```python
from build123d import *

# Parameters (mm, degrees)
SKETCH_W     = 33
SKETCH_H     = 50
SKETCH_R     = 3.25
PAD_DEPTH    = 3
FILLET_R     = 2
FILLET001_R  = 10
PAD001_DEPTH = 4.8
SKETCH002_R  = 1.25
POCKET_DEPTH = 8.001
CHAMFER_SIZE = 0.5


with BuildPart() as part:
    # Sketch → Pad (new body)
    with BuildSketch(Plane.XY):
        with Locations((16.5, 25)):
            Rectangle(SKETCH_W, SKETCH_H)
        with Locations((24, 41)):
            Circle(SKETCH_R, mode=Mode.SUBTRACT)
    extrude(amount=PAD_DEPTH)

    # Fillet
    fillet_edges = [part.edges().sort_by_distance(p)[0] for p in [
        (0, 0, 1.5),
    ]]
    fillet(fillet_edges, radius=FILLET_R)

    # Fillet001
    fillet001_edges = [part.edges().sort_by_distance(p)[0] for p in [
        (33, 0, 1.5),
        (0, 50, 1.5),
        (33, 50, 1.5),
    ]]
    fillet(fillet001_edges, radius=FILLET001_R)

    # Sketch001 → Pad001 (join)
    with BuildSketch(Plane.XY.offset(3)):
        Polygon((20, 22), (20, 27.5), (1, 27.5), (1, 22), (17, 22), (17, 21), (20, 21), align=None)
        Polygon((1, 0.5), (1, 6), (17, 6), (17, 7), (20, 7), (20, 6), (20, 0.5), align=None)
    extrude(amount=PAD001_DEPTH)

    # Sketch002 → Pocket (cut, through all)
    with BuildSketch(Plane.XY.offset(8)):
        with Locations((16, 24)):
            Circle(SKETCH002_R)
        with Locations((16, 4)):
            Circle(SKETCH002_R)
    extrude(amount=-POCKET_DEPTH, mode=Mode.SUBTRACT)

    # Chamfer
    chamfer_edges = [part.edges().sort_by_distance(p)[0] for p in [
        (9, 22, 7.8),
        (9, 6, 7.8),
        (17, 21.5, 7.8),
        (17, 6.5, 7.8),
        (18.5, 7, 7.8),
        (18.5, 21, 7.8),
    ]]
    chamfer(chamfer_edges, length=CHAMFER_SIZE)


solid = part.part
```
Can you work these out from the model? Positions are in its coordinate system, mm. A direction names the side the tool comes from. Coordinates: 2 decimals unless noted, no trailing zeros. Write each loop counter-clockwise with the first axis right and the second up, starting at its lowest first coordinate (ties: lowest second). Pieces come first, ordered by that corner, then holes. Notation, with made-up numbers: M -3.75,60 L 3.25,60 A22 ccw 3.25,97 Z; hole C 16,36 d11. An arc over 180 degrees is marked long. Answer as CSV lines item,"result".
Item 1: We'd pull the mould along X, two halves only. Please class faces 1 (the cylindrical face through (15.73, 2.78, 3.95)), 2 (the flat face through (0, 21, 1)), 3 (the cylindrical face through (29.99, 47.15, 1.52)): +X half, -X half, draft (parallel to the pull), parting line (faces both ways), or undercut.
Geometry results:
face 1,"undercut"
face 2,"-X half"
face 3,"+X half"
Item 2: Imagine slicing it at A-A on z = 5.25. List the corners of the cut face in (x, y) for me, plus the area to 3 significant figures.
Geometry results:
outline,"M 1,0.5 L 20,0.5 L 20,7 L 17,7 L 17,6 L 1,6 Z; M 1,22 L 17,22 L 17,21 L 20,21 L 20,27.5 L 1,27.5 Z; hole C 16,4 d2.5; hole C 16,24 d2.5"
area,"205 mm2"
Item 3: I'm going to push flat-ended pins straight in: P1, Ø2.5, axis at x = 18, z = 4.5, coming from the +Y side; P2, Ø0.5, axis at y = 6.5, z = 6, coming from the -X side; P3, Ø2.5, axis at y = 25.5, z = 4.5, coming from the +X side; P4, Ø4, axis at x = 24, y = 41, coming from the +Z side. Where does each tip first touch, or does it pass through?
Geometry results:
P1,"stops at y = 27.5"
P2,"stops at x = 17"
P3,"stops at x = 20"
P4,"passes through"
Item 4: Imagine slicing it at C-C on y = 41. List the corners of the cut face in (x, z) for me, plus the area to 3 significant figures.
Geometry results:
outline,"M 0.05,0 L 20.75,0 L 20.75,3 L 0.05,3 Z; M 27.25,0 L 32.95,0 L 32.95,3 L 27.25,3 Z"
area,"79.2 mm2"
Item 5: Imagine slicing it at D-D on x = 24. List the corners of the cut face in (y, z) for me.
Geometry results:
outline,"M 0.05,0 L 37.75,0 L 37.75,3 L 0.05,3 Z; M 44.25,0 L 49.95,0 L 49.95,3 L 44.25,3 Z"
Item 6: On a 3-axis mill with a long thin cutter (end or side, diameter ignored), from which of +Z, -Z, +X, -X, +Y, -Y can I reach the whole of each face in a straight line? I mean faces 4 (the flat face through (20, 4, 5)), 5 (the flat face through (1, 25, 5)), 6 (the flat face through (9, 22, 5)), 7 (the flat face through (11, 27.5, 5)), 8 (the flat face through (18, 7, 5)). Say none if no direction works.
Geometry results:
face 4,"+Z, +X, +Y, -Y"
face 5,"+Z, -X, +Y, -Y"
face 6,"+Z, -X"
face 7,"+Z, +X, -X, +Y"
face 8,"+Z, +X, -X"
Item 7: Imagine slicing it at B-B on x = 16. List the corners of the cut face in (y, z) for me.
Geometry results:
outline,"M 0,0 L 2.75,0 L 2.75,7.8 L 0.5,7.8 L 0.5,3 L 0,3 Z; M 5.25,0 L 22.75,0 L 22.75,7.8 L 22.5,7.8 L 22,7.3 L 22,3 L 6,3 L 6,7.3 L 5.5,7.8 L 5.25,7.8 Z; M 25.25,0 L 50,0 L 50,3 L 27.5,3 L 27.5,7.8 L 25.25,7.8 Z"
Item 8: Please list where these lines run through material, in increasing order: line 1 along Y through (x, z) = (16, 5.25); line 2 along Y through (x, z) = (16, 2); line 3 along Z through (x, y) = (4, 9.5).
Geometry results:
line 1,"y = 0.5 to 2.75, 5.25 to 6, 22 to 22.75, 25.25 to 27.5"
line 2,"y = 0 to 2.75, 5.25 to 22.75, 25.25 to 50"
line 3,"z = 0 to 3"
